Design review of the part built by this model. Coordinates are the model's own, in mm. A direction names the side the tool comes from. Round coordinates to 2 decimals unless told otherwise and drop trailing zeros. Order: outer loops, then holes, each group sorted by start corner. A loop starts at its lowest first (then second) coordinate and runs counter-clockwise, first axis right, second up. Notation, with made-up numbers: M -39,39 L -13,39 A20 ccw -13,58 Z; hole C 36,89 d8. An arc over 180 degrees is marked long. Use a Markdown table: item, result. Add a question column.
(1) For pin 1 (8 mm diameter, centred on y = 0, z = 23, fed in from +X); pin 2 (8 mm diameter, centred on x = -201.5, y = 8.5, fed in from -Z); pin 3 (6 mm diameter, centred on x = -196, z = 23, fed in from -Y); pin 4 (10 mm diameter, centred on x = -47, y = 12, fed in from -Z), all flat-tipped, find the tip position at first contact; note any pin that passes through.
(2) Machinability: for faces 5 (the face through (11.5, 1.3, -11.5)), 6 (the face through (-126, 0, 18)), 7 (the face through (7.06, -9.86, 11.64)), which of the approach directions +Z, -Z, +X, -X, +Y, -Y give a long, thin tool a straight path to every point of the face, cutting with its end or side? Answer none if there is none.
(3) Take a section at A-A (x = -151.5). Write out the cut boundary in (y, z), then the cut area to 3 significant figures.
(4) To check wall thickness, follow probe 1 along Y at (x, z) = (9.75, -10); probe 2 along Z at (x, y) = (-182, -0.5); probe 3 along X at (y, z) = (3.5, 6). State the ranges of each line that lie inside material, in increasing order. Write a range as from..to.
(5) The part is to be moulded in two halves that separate along X. For faces 1 (the face through (7, 0, 32.5)), 2 (the face through (9.929, -3.441, 20.806)), 3 (the face through (-163.95, 3.4, 0.1)), 4 (the face through (-171.95, 0, 0)), say which applies: released by +X, released by -X, zero draft, split by the parting line, or undercut.
Autodesk Inventor part; units mm, degrees
ref_plane "HUELSE3_1_XY" through (11, 1.4, -14) normal (1, 0, 0) x (0, 0, -1)
ref_plane "HUELSE3_1_YZ" through (11, 1.4, -14) normal (0, 0, -1) x (0, 1, 0)
ref_plane "HUELSE3_1_ZX" through (11, 1.4, -14) normal (0, 1, 0) x (1, 0, 0)
sketch "Skizze_1" plane through (12, 0, 0) normal (1, 0, 0) x (0, 0, -1)
  line L0 (-32.5, -14) -> (-31.5, -15)
  line L1 (-31.5, -15) -> (31.5, -15)
  line L2 (31.5, -15) -> (32.5, -14)
  line L3 (32.5, -14) -> (32.5, 14)
  line L4 (32.5, 14) -> (31.5, 15)
  line L5 (31.5, 15) -> (-31.5, 15)
  line L6 (-31.5, 15) -> (-32.5, 14)
  line L7 (-32.5, 14) -> (-32.5, -14)
extrude "Extrusion1" add sketch "Skizze_1" against normal blind 10
sketch "Skizze_2" plane through (0, 0, 0) normal (0, 1, 0) x (1, 0, 0)
  line L0 (-252, -23) -> (2, -23)
  line L1 (2, -23) -> (2, -28)
  line L2 (2, -28) -> (-251, -28)
  line L3 (-251, -28) -> (-252, -27.4226)
  line L4 (-252, -27.4226) -> (-252, -23)
  line L5 (-252, -23) -> (2, -23)
sketch "Skizze_3" plane through (0, 0, 0) normal (0, 1, 0) x (1, 0, 0)
  line L0 (-252, 23) -> (2, 23)
  line L1 (2, 23) -> (2, 18)
  line L2 (2, 18) -> (-251, 18)
  line L3 (-251, 18) -> (-252, 18.5774)
  line L4 (-252, 18.5774) -> (-252, 23)
  line L5 (-252, 23) -> (2, 23)
sketch "Skizze_4" plane through (0, -8.6, 0) normal (0, 1, 0) x (1, 0, 0)
  line L0 (12, -10) -> (2, -10)
  line L1 (2, -10) -> (2, -7.5)
  line L2 (2, -7.5) -> (2.433, -7.933)
  line L3 (2.433, -7.933) -> (11.567, -7.933)
  line L4 (11.567, -7.933) -> (12, -7.5)
  line L5 (12, -7.5) -> (12, -10)
  line L6 (12, -10) -> (2, -10)
revolve "Revolution1" cut sketch "Skizze_4" angle 360 about axis through (12, -8.6, 10) along (1, 0, 0)
thread "Thread1"
sketch "Skizze_5" plane through (0, -8.6, 0) normal (0, 1, 0) x (1, 0, 0)
  line L0 (12, 10) -> (2, 10)
  line L1 (2, 10) -> (2, 12.5)
  line L2 (2, 12.5) -> (2.433, 12.067)
  line L3 (2.433, 12.067) -> (11.567, 12.067)
  line L4 (11.567, 12.067) -> (12, 12.5)
  line L5 (12, 12.5) -> (12, 10)
  line L6 (12, 10) -> (2, 10)
revolve "Revolution2" cut sketch "Skizze_5" angle 360 about axis through (12, -8.6, -10) along (1, 0, 0)
thread "Thread2"
sketch "Skizze_6" plane through (0, 11.4, 0) normal (0, 1, 0) x (1, 0, 0)
  line L0 (12, -10) -> (2, -10)
  line L1 (2, -10) -> (2, -7.5)
  line L2 (2, -7.5) -> (2.433, -7.933)
  line L3 (2.433, -7.933) -> (11.567, -7.933)
  line L4 (11.567, -7.933) -> (12, -7.5)
  line L5 (12, -7.5) -> (12, -10)
  line L6 (12, -10) -> (2, -10)
revolve "Revolution3" cut sketch "Skizze_6" angle 360 about axis through (12, 11.4, 10) along (1, 0, 0)
thread "Thread3"
sketch "Skizze_7" plane through (0, 11.4, 0) normal (0, 1, 0) x (1, 0, 0)
  line L0 (12, 10) -> (2, 10)
  line L1 (2, 10) -> (2, 12.5)
  line L2 (2, 12.5) -> (2.433, 12.067)
  line L3 (2.433, 12.067) -> (11.567, 12.067)
  line L4 (11.567, 12.067) -> (12, 12.5)
  line L5 (12, 12.5) -> (12, 10)
  line L6 (12, 10) -> (2, 10)
revolve "Revolution4" cut sketch "Skizze_7" angle 360 about axis through (12, 11.4, -10) along (1, 0, 0)
thread "Thread4"
sketch "Skizze_8" plane through (0, 0, 0) normal (0, 0, 1) x (1, 0, 0)
  line L0 (2, 0) -> (-171.95, 0)
  line L1 (-171.95, 0) -> (-171.95, 8)
  line L2 (-171.95, 8) -> (-163.95, 8)
  line L3 (-163.95, 8) -> (-163.95, 3)
  line L4 (-163.95, 3) -> (2, 3)
  line L5 (2, 3) -> (2, 0)
  line L6 (2, 0) -> (-171.95, 0)
revolve "Revolution5" add sketch "Skizze_8" angle 360 about axis through (2, 0, 0) along (1, 0, 0)
sketch "Sketch9" plane through (12, 15, 31.5) normal (0, 1, 0) x (1, 0, 0)
  point P0 (-5, 8.5)
hole "Hole1" at (7, 15, 23) direction (0, -1, 0) diameter 3.242 depth 15 countersink diameter 4 countersink angle 90
sketch "Sketch10" plane through (12, 15, 31.5) normal (0, 1, 0) x (1, 0, 0)
  point P0 (-5, 54.5)
hole "Hole2" at (7, 15, -23) direction (0, -1, 0) diameter 3.242 depth 15 countersink diameter 4 countersink angle 90
revolve "Revolution6" add sketch "Skizze_2" angle 360 about axis through (-252, 0, 23) along (-1, 0, 0)
revolve "Revolution7" add sketch "Skizze_3" angle 360 about axis through (-252, 0, -23) along (-1, 0, 0)
sketch "Sketch11" plane through (12, 0, 0) normal (1, 0, 0) x (0, 0, -1)
  point P0 (14, 1.4)
hole "Hole3" at (12, 1.4, -14) direction (-1, 0, 0) diameter 5 depth 1 tip angle 120
sketch "Sketch12" plane through (12, 0, 0) normal (1, 0, 0) x (0, 0, -1)
  point P0 (-14, 1.4)
hole "Hole4" at (12, 1.4, 14) direction (-1, 0, 0) diameter 5 depth 1 tip angle 120
sketch "Sketch_4" plane through (0, 0, 0) normal (0, 1, 0) x (1, 0, 0)
  line L0 (12, 23) -> (11.65, 23)
  line L1 (11.65, 23) -> (11.65, 26.4725)
  arc A0 (11.65, 26.4725) -> (11.1936, 26.9706) centre (11.15, 26.4725) ccw
  line L2 (11.1936, 26.9706) -> (8, 27.25)
  line L3 (8, 27.25) -> (8, 28)
  line L4 (8, 28) -> (12, 28)
  line L5 (12, 28) -> (12, 23)
  line L6 (12, 23) -> (11.65, 23)
revolve "Revolution8" cut sketch "Sketch_4" angle 360 about axis through (12, 0, -23) along (1, 0, 0)
sketch "Sketch_6" plane through (0, 0, 0) normal (0, 1, 0) x (1, 0, 0)
  line L0 (12, -23) -> (11.65, -23)
  line L1 (11.65, -23) -> (11.65, -19.5275)
  arc A0 (11.65, -19.5275) -> (11.1936, -19.0294) centre (11.15, -19.5275) ccw
  line L2 (11.1936, -19.0294) -> (8, -18.75)
  line L3 (8, -18.75) -> (8, -18)
  line L4 (8, -18) -> (12, -18)
  line L5 (12, -18) -> (12, -23)
  line L6 (12, -23) -> (11.65, -23)
revolve "Revolution9" cut sketch "Sketch_6" angle 360 about axis through (12, 0, 23) along (1, 0, 0)
sketch "Sketch_7" plane through (11.65, 0, 23) normal (1, 0, 0) x (0, 0, -1)
  arc A0 (-1.8677, -0.5727) -> (-1.4298, -1.3311) centre (-1.5588, -0.9) ccw
  arc A1 (-0.4379, -1.9038) -> (-1.4298, -1.3311) centre (-1.2041, -2.0855) ccw
  arc A2 (-0.4379, -1.9038) -> (0.4379, -1.9038) centre (0, -1.8) ccw
  arc A3 (1.4298, -1.3311) -> (0.4379, -1.9038) centre (1.2041, -2.0855) ccw
  arc A4 (1.4298, -1.3311) -> (1.8677, -0.5727) centre (1.5588, -0.9) ccw
  arc A5 (1.8677, 0.5727) -> (1.8677, -0.5727) centre (2.4082, 0) ccw
  arc A6 (1.8677, 0.5727) -> (1.4298, 1.3311) centre (1.5588, 0.9) ccw
  arc A7 (0.4379, 1.9038) -> (1.4298, 1.3311) centre (1.2041, 2.0855) ccw
  arc A8 (0.4379, 1.9038) -> (-0.4379, 1.9038) centre (0, 1.8) ccw
  arc A9 (-1.4298, 1.3311) -> (-0.4379, 1.9038) centre (-1.2041, 2.0855) ccw
  arc A10 (-1.4298, 1.3311) -> (-1.8677, 0.5727) centre (-1.5588, 0.9) ccw
  arc A11 (-1.8677, -0.5727) -> (-1.8677, 0.5727) centre (-2.4082, 0) ccw
extrude "Extrusion2" cut sketch "Sketch_7" against normal blind 2.48
sketch "Sketch_8" plane through (11.65, 0, -23) normal (1, 0, 0) x (0, 0, -1)
  arc A0 (-1.8677, -0.5727) -> (-1.4298, -1.3311) centre (-1.5588, -0.9) ccw
  arc A1 (-0.4379, -1.9038) -> (-1.4298, -1.3311) centre (-1.2041, -2.0855) ccw
  arc A2 (-0.4379, -1.9038) -> (0.4379, -1.9038) centre (0, -1.8) ccw
  arc A3 (1.4298, -1.3311) -> (0.4379, -1.9038) centre (1.2041, -2.0855) ccw
  arc A4 (1.4298, -1.3311) -> (1.8677, -0.5727) centre (1.5588, -0.9) ccw
  arc A5 (1.8677, 0.5727) -> (1.8677, -0.5727) centre (2.4082, 0) ccw
  arc A6 (1.8677, 0.5727) -> (1.4298, 1.3311) centre (1.5588, 0.9) ccw
  arc A7 (0.4379, 1.9038) -> (1.4298, 1.3311) centre (1.2041, 2.0855) ccw
  arc A8 (0.4379, 1.9038) -> (-0.4379, 1.9038) centre (0, 1.8) ccw
  arc A9 (-1.4298, 1.3311) -> (-0.4379, 1.9038) centre (-1.2041, 2.0855) ccw
  arc A10 (-1.4298, 1.3311) -> (-1.8677, 0.5727) centre (-1.5588, 0.9) ccw
  arc A11 (-1.8677, -0.5727) -> (-1.8677, 0.5727) centre (-2.4082, 0) ccw
extrude "Extrusion3" cut sketch "Sketch_8" against normal blind 2.48
sketch "Sketch_9" plane through (0, 0, 0) normal (0, 0, 1) x (1, 0, 0)
  line L0 (12, 0) -> (9.868, 0)
  line L1 (9.868, 0) -> (11.6, 1.732)
  line L2 (11.6, 1.732) -> (11.6, 3.1)
  arc A0 (11.6, 3.1) -> (11.2, 3.5) centre (11.2, 3.1) ccw
  line L3 (11.2, 3.5) -> (7.6, 3.5)
  line L4 (7.6, 3.5) -> (7.6, 4)
  line L5 (7.6, 4) -> (12, 4)
  line L6 (12, 4) -> (12, 0)
  line L7 (12, 0) -> (9.868, 0)
revolve "Revolution10" cut sketch "Sketch_9" angle 360 about axis through (12, 0, 0) along (1, 0, 0)
sketch "Sketch_10" plane through (11.6, 0, 0) normal (1, 0, 0) x (0, 1, 0)
  line L0 (-1.5, -0.866) -> (0, -1.7321)
  line L1 (0, -1.7321) -> (1.5, -0.866)
  line L2 (1.5, -0.866) -> (1.5, 0.866)
  line L3 (1.5, 0.866) -> (0, 1.7321)
  line L4 (0, 1.7321) -> (-1.5, 0.866)
  line L5 (-1.5, 0.866) -> (-1.5, -0.866)
extrude "Extrusion4" cut sketch "Sketch_10" against normal blind 2
ref_plane "HUELSE3_1_XY" through (11, 1.4, -14) normal (1, 0, 0) x (0, 0, -1)
ref_plane "HUELSE3_1_YZ" through (11, 1.4, -14) normal (0, 0, -1) x (0, 1, 0)
ref_plane "HUELSE3_1_ZX" through (11, 1.4, -14) normal (0, 1, 0) x (1, 0, 0)
ref_plane "HUELSE3_2_XY" through (11, 1.4, 14) normal (1, 0, 0) x (0, 0, -1)
ref_plane "HUELSE3_2_YZ" through (11, 1.4, 14) normal (0, 0, -1) x (0, 1, 0)
ref_plane "HUELSE3_2_ZX" through (11, 1.4, 14) normal (0, 1, 0) x (1, 0, 0)
ref_plane "kolben_dfm_XY" through (0, 0, 0) normal (-1, 0, 0) x (0, 0, -1)
ref_plane "kolben_dfm_YZ" through (0, 0, 0) normal (0, 0, -1) x (0, -1, 0)
ref_plane "kolben_dfm_ZX" through (0, 0, 0) normal (0, -1, 0) x (-1, 0, 0)
properties part number "529120 DFM-16-150-B-P-A-KF---(K)"
Verdict:
| question | item | result |
|---|---|---|
| 1 | pin 1 | stops at x = 11.65 |
| 1 | pin 2 | stops at z = -25.18 |
| 1 | pin 3 | stops at y = -5 |
| 1 | pin 4 | passes through |
| 2 | face 5 | +X |
| 2 | face 6 | -X |
| 2 | face 7 | +X, -X |
| 3 | outline | C 0,-23 d10; C 0,23 d10; C 0,0 d6 |
| 3 | area | 185 mm^2 |
| 4 | probe 1 | y = -15..-10.67, -6.53..9.33, 13.47..15 |
| 4 | probe 2 | z = -27.97..-18.03, 18.03..27.97 |
| 4 | probe 3 | x = -171.95..-163.95, 2..12 |
| 5 | face 1 | zero draft |
| 5 | face 2 | released by +X |
| 5 | face 3 | undercut |
| 5 | face 4 | released by -X |
